from build123d import *

# Parameters (mm, degrees)
F1_DEPTH = 6
F3_DEPTH = 2
F4_R     = 2.25
F5_DEPTH = 8.001
F6_R     = 3.75
F7_DEPTH = 2
F9_DEPTH = 6
F10_SIZE = 3


with BuildPart() as f1:
    # F0 (on Top) → F1 (new body)
    with BuildSketch(Plane.XY):
        Polygon((-30, 0), (-10, 0), (-10, -40), (0, -40), (10, -40), (10, 0), (30, 0), (30, 20), (0, 20), (-30, 20), align=None)
    extrude(amount=F1_DEPTH)

    # F2 (on face) → F3 (join)
    with BuildSketch(Plane.XY.offset(6)):
        Polygon((2.71, 0), (0, 0), (-2.71, 0), (-2.71, -40), (2.71, -40), align=None)
        Polygon((30, 7.29), (30, 12.71), (-30, 12.71), (-30, 10), (-30, 7.29), align=None)
    extrude(amount=F3_DEPTH)

    # F4 (on face) → F5 (cut, through all)
    with BuildSketch(Plane(origin=(0, 0, 0), x_dir=(1, 0, 0), z_dir=(0, 0, -1))):
        with Locations((-20, -10)):
            Circle(F4_R)
        with Locations((0, 10)):
            Circle(F4_R)
        with Locations((0, 30)):
            Circle(F4_R)
        with Locations((20.741304, -10)):
            Circle(F4_R)
        with Locations((0, -10)):
            Circle(F4_R)
    extrude(amount=-F5_DEPTH, mode=Mode.SUBTRACT)

    # F6 (on face) → F7 (cut)
    with BuildSketch(Plane(origin=(0, 0, 0), x_dir=(1, 0, 0), z_dir=(0, 0, -1))):
        with Locations((0, 30)):
            Circle(F6_R)
        with Locations((0, 10)):
            Circle(F6_R)
        with Locations((20.741304, -10)):
            Circle(F6_R)
        with Locations((-20, -10)):
            Circle(F6_R)
        with Locations((0, -10)):
            Circle(F6_R)
    extrude(amount=-F7_DEPTH, mode=Mode.SUBTRACT)

    # F8 (on face) → F9 (join)
    with BuildSketch(Plane(origin=(0, 0, 0), x_dir=(1, 0, 0), z_dir=(0, 0, -1))):
        Polygon((-10, 0), (-10, 40), (-30, 0), align=None)
        Polygon((30, 0), (10, 40), (10, 0), align=None)
    extrude(amount=-F9_DEPTH)

    # F10
    f10_edges = [f1.edges().sort_by_distance(p)[0] for p in [
        (0, -40, 0),
        (-20, -20, 0),
        (20, -20, 0),
        (30, 10, 0),
        (0, 20, 0),
        (-30, 10, 0),
    ]]
    chamfer(f10_edges, length=F10_SIZE)


solid = f1.part
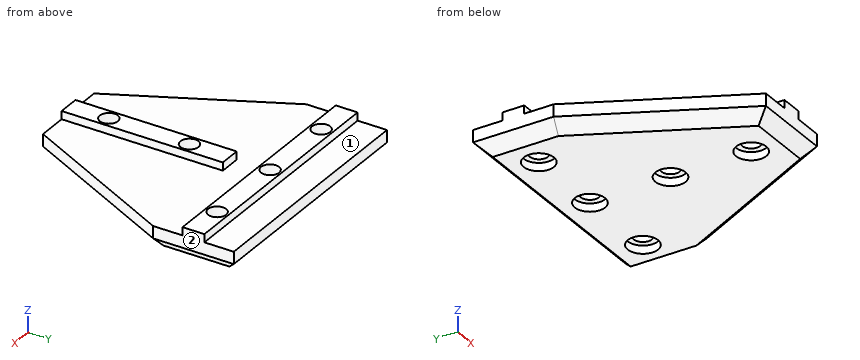
Work out the finished part from the listing and answer in its coordinate system (mm). Face numbers are marked on the shaded views. A direction names the side the tool comes from. Give positions to 0.01 mm unless a question says otherwise; leave off trailing zeros. Write each loop counter-clockwise with the first axis right and the second up, starting at its lowest first coordinate (ties: lowest second). Pieces come first, ordered by that corner, then holes.
Q1. Straight lines are drawn through the part: L1, parallel to X at y = 10, z = 4.3; L2, parallel to Y at x = 0, z = 0.5; L3, parallel to Y at x = 0, z = 0.55. For each, find the intervals that lie inside material, in ascending order.
Answer:
L1: x = -30 to -22.25, -17.75 to -2.25, 2.25 to 18.49, 22.99 to 30
L2: y = -37.5 to -33.75, -26.25 to -13.75, -6.25 to 6.25, 13.75 to 17.5
L3: y = -37.55 to -33.75, -26.25 to -13.75, -6.25 to 6.25, 13.75 to 17.55
Q2. Given pin 1 (6 mm diameter, centred on x = 0, y = -29.5, fed in from -Z); pin 2 (1.5 mm diameter, centred on y = -27, z = 6.5, fed in from -X); pin 3 (0.6 mm diameter, centred on x = 5.5, z = 7, fed in from -Y), each flat-ended and moving along its own axis, determine where each tip first touches the part or whether it passes through.
Answer:
pin 1: stops at z = 2
pin 2: stops at x = -16.78
pin 3: stops at y = 7.29
Q3. The part is cut by section B-B on y = -30. Give the vertices of the cut face in (x, z), and give its area (3 significant figures).
Answer:
outline: (-15, 3) - (-11.65, 0) - (-3.75, 0) - (-3.75, 2) - (-2.25, 2) - (-2.25, 8) - (-2.71, 8) - (-2.71, 6) - (-15, 6) - close; (2.25, 2) - (3.75, 2) - (3.75, 0) - (11.65, 0) - (15, 3) - (15, 6) - (2.71, 6) - (2.71, 8) - (2.25, 8) - close
area: 139 mm2
Q4. The part is cut by section A-A on y = 10. State how many separate pieces and enclosed holes the cut face has, and give its area (3 significant figures).
Answer:
separate pieces: 4
enclosed holes: 0
area: 345 mm2
Q5. The part is cut by section C-C on x = -20. Give the vertices of the cut face in (y, z).
Answer:
outline: (-20, 3) - (-13.29, 0) - (6.25, 0) - (6.25, 2) - (7.75, 2) - (7.75, 8) - (7.29, 8) - (7.29, 6) - (-20, 6) - close; (12.25, 2) - (13.75, 2) - (13.75, 0) - (17, 0) - (20, 3) - (20, 6) - (12.71, 6) - (12.71, 8) - (12.25, 8) - close
Q6. A tool of negligible diameter and unlimited length cuts with its end or side. For the marked faces 1 and 2, from which of +Z, -Z, +X, -X, +Y, -Y can it reach the whole face along a straight path? Write none if from no direction.
Answer:
face 1: +Z, +X, -X, +Y
face 2: +Z, -Z, +X, +Y, -Y
